Geometry: final body of the model. Coordinates: model frame, mm. Face numbers are marked on the shaded views. A direction names the side the tool comes from. Give positions to 0.01 mm unless a question says otherwise; leave off trailing zeros. Write each loop counter-clockwise with the first axis right and the second up, starting at its lowest first coordinate (ties: lowest second). Pieces come first, ordered by that corner, then holes. Notation, with made-up numbers: (67.25, -34.75) -> (122.25, -34.75) arc R19 cw to (122.25, -14.75) -> close; hole circle Ø5 at (57, 22). An arc over 180 degrees is marked (long way). Answer in a Markdown table with one row per item. Add a question column.
Item 1: Section query B-B on z = 33. Output: boundary loops of the cut face in (x, y).
Item 2: Access query for the marked faces 1, 2 and 3. Directions: +Z, -Z, +X, -X, +Y, -Y. A direction counts if a zero-diameter tool reaches every point of the face in a straight line with its end or side. Return the directions, or none.
Item 3: Section query D-D on z = -75.5. Output: boundary loops of the cut face in (x, y), plus the area to 3 significant figures.
Item 4: Section query A-A on x = 117. Output: boundary loops of the cut face in (y, z).
Item 5: Material intervals for probe 1 along Z at (x, y) = (72, 23); probe 2 along X at (y, z) = (17.5, -63); probe 3 along Y at (x, z) = (-121.5, -13), sorted ascending. Write a range as from..to.
Item 6: First-contact query: P1, Ø10, axis at y = 18.5, z = -2, coming from the +X side; P2, Ø5, axis at y = 19.5, z = -35, coming from the +X side; P3, Ø10, axis at y = 13, z = -11.5, coming from the -X side. Flat tips, straight axial feed; report the tip coordinate or a pass-through.
Item 7: Section query C-C on y = 13.5. State how many separate pieces and enclosed holes the cut face has, plus the area to 3 significant figures.
```python
from build123d import *

# Parameters (mm, degrees)
BOSS_EXTRUDE1_DEPTH = 5
SKETCH2_W           = 71.143127042
SKETCH2_H           = 10
BOSS_EXTRUDE3_DEPTH = 25
SKETCH3_W           = 10
SKETCH3_H           = 10
BOSS_EXTRUDE4_DEPTH = 25
BOSS_EXTRUDE5_DEPTH = 10
SKETCH6_W           = 10
SKETCH6_H           = 60
BOSS_EXTRUDE6_DEPTH = 25
BOSS_EXTRUDE7_DEPTH = 10
SKETCH9_W           = 97.713745916
SKETCH9_H           = 10
BOSS_EXTRUDE8_DEPTH = 25
SKETCH11_R          = 2.5
CUT_EXTRUDE1_DEPTH  = 5
SKETCH12_R          = 1.788924299
CUT_EXTRUDE2_DEPTH  = 10


with BuildPart() as part:
    # Sketch1 → Boss-Extrude1 (new body)
    with BuildSketch(Plane(origin=(0, 0, 0), x_dir=(1, 0, 0), z_dir=(0, 1, 0))):
        with BuildLine():
            Line((-130, 90), (130, 90))
            ThreePointArc((130, 90), (151.213203436, 81.213203436), (160, 60))
            Line((160, 60), (160, -60))
            ThreePointArc((160, -60), (151.213203436, -81.213203436), (130, -90))
            Line((130, -90), (-130, -90))
            ThreePointArc((-130, -90), (-151.213203436, -81.213203436), (-160, -60))
            Line((-160, -60), (-160, 60))
            ThreePointArc((-160, 60), (-151.213203436, 81.213203436), (-130, 90))
        make_face()
    extrude(amount=BOSS_EXTRUDE1_DEPTH)

    # Sketch2 → Boss-Extrude3 (add)
    with BuildSketch(Plane(origin=(0, 5, 0), x_dir=(1, 0, 0), z_dir=(0, 1, 0))):
        with Locations((-84.428436479, 65)):
            Rectangle(SKETCH2_W, SKETCH2_H)
        with Locations((84.428436479, 65)):
            Rectangle(SKETCH2_W, SKETCH2_H)
        with Locations((84.428436479, -65)):
            Rectangle(SKETCH2_W, SKETCH2_H)
        with Locations((-84.428436479, -65)):
            Rectangle(SKETCH2_W, SKETCH2_H)
    extrude(amount=BOSS_EXTRUDE3_DEPTH)

    # Sketch3 → Boss-Extrude4 (add)
    with BuildSketch(Plane(origin=(0, 5, 0), x_dir=(1, 0, 0), z_dir=(0, 1, 0))):
        with Locations((-140, -5)):
            Rectangle(SKETCH3_W, SKETCH3_H)
    boss_extrude4 = extrude(amount=BOSS_EXTRUDE4_DEPTH)

    # Sketch5 → Boss-Extrude5 (add)
    with BuildSketch(Plane(origin=(0, 0, 0), x_dir=(-1, 0, 0), z_dir=(0, 0, -1))):
        Polygon((145, 5), (145, 30), (160, 5), align=None)
    boss_extrude5 = extrude(amount=-BOSS_EXTRUDE5_DEPTH)

    # Sketch6 → Boss-Extrude6 (add)
    with BuildSketch(Plane(origin=(0, 5, 0), x_dir=(1, 0, 0), z_dir=(0, 1, 0))):
        with Locations((70, 0)):
            Rectangle(SKETCH6_W, SKETCH6_H)
    extrude(amount=BOSS_EXTRUDE6_DEPTH)

    # Sketch8 → Boss-Extrude7 (add)
    with BuildSketch(Plane.XY.offset(30)):
        Polygon((75, 30), (88.085238775, 5), (75, 5), align=None)
    boss_extrude7 = extrude(amount=-BOSS_EXTRUDE7_DEPTH)

    # Mirror1: Boss-Extrude7 across plane
    add(boss_extrude7.mirror(Plane(origin=(0, 0, 0), x_dir=(1, 0, 0), z_dir=(0, 0, -1))))

    # Mirror2: Boss-Extrude4, Boss-Extrude5 across plane
    add(boss_extrude4.mirror(Plane(origin=(-145, 30, 0), x_dir=(1, 0, 0), z_dir=(0, 0, 1))))
    add(boss_extrude5.mirror(Plane(origin=(-145, 30, 0), x_dir=(1, 0, 0), z_dir=(0, 0, 1))))

    # Sketch9 → Boss-Extrude8 (add)
    with BuildSketch(Plane(origin=(0, 5, 0), x_dir=(1, 0, 0), z_dir=(0, 1, 0))):
        with Locations((0, -35)):
            Rectangle(SKETCH9_W, SKETCH9_H)
    boss_extrude8 = extrude(amount=BOSS_EXTRUDE8_DEPTH)

    # Mirror3: Boss-Extrude8 across plane
    add(boss_extrude8.mirror(Plane(origin=(0, 0, 0), x_dir=(1, 0, 0), z_dir=(0, 0, -1))))

    # Sketch11 → Cut-Extrude1 (cut)
    with BuildSketch(Plane(origin=(0, 5, 0), x_dir=(1, 0, 0), z_dir=(0, 1, 0))):
        with Locations(Location((-118.275690488, 50, 0), (0, 0, 270))):
            Circle(SKETCH11_R)
        with Locations(Location((-118.275690488, -50, 0), (0, 0, 270))):
            Circle(SKETCH11_R)
        with Locations(Location((20.561944572, -50, 0), (0, 0, 270))):
            Circle(SKETCH11_R)
        with Locations(Location((20.561944572, 50, 0), (0, 0, 270))):
            Circle(SKETCH11_R)
    extrude(amount=-CUT_EXTRUDE1_DEPTH, mode=Mode.SUBTRACT)

    # Sketch12 → Cut-Extrude2 (cut)
    with BuildSketch(Plane.XY.offset(70)):
        with Locations((-58.856872958, 27)):
            Circle(SKETCH12_R)
        with Locations(Location((-58.856872958, 8, 0), (0, 0, 180))):
            Circle(SKETCH12_R)
        with Locations((58.856872958, 8)):
            Circle(SKETCH12_R)
        with Locations(Location((58.856872958, 27, 0), (0, 0, 180))):
            Circle(SKETCH12_R)
    cut_extrude2 = extrude(amount=-CUT_EXTRUDE2_DEPTH, mode=Mode.SUBTRACT)

    # Mirror4: Cut-Extrude2 across plane
    add(cut_extrude2.mirror(Plane.XY), mode=Mode.SUBTRACT)


solid = part.part
```
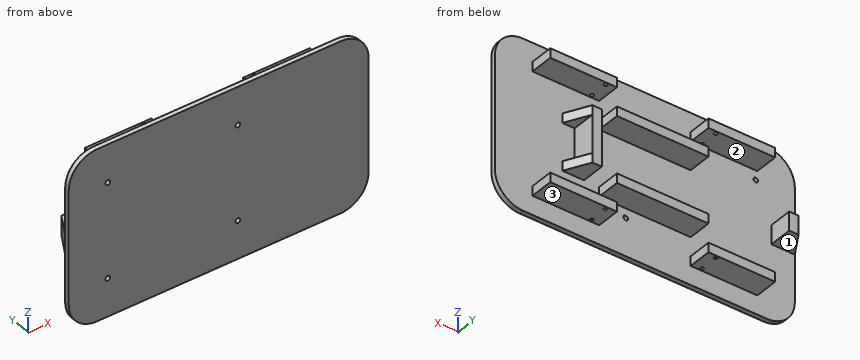
Findings below:
| question | item | result |
|---|---|---|
| 1 | outline | (-160, 0) -> (160, 0) -> (160, 5) -> (48.86, 5) -> (48.86, 30) -> (-48.86, 30) -> (-48.86, 5) -> (-160, 5) -> close |
| 2 | face 1 | -Z, -X, +Y |
| 2 | face 2 | +X, -X, +Y |
| 2 | face 3 | -Z, +X, -X, +Y |
| 3 | outline | (-155.69, 0) -> (155.69, 0) -> (155.69, 5) -> (-155.69, 5) -> close |
| 3 | area | 1,560 mm^2 |
| 4 | outline | (0, -90) -> (5, -90) -> (5, -70) -> (30, -70) -> (30, -60) -> (5, -60) -> (5, 60) -> (30, 60) -> (30, 70) -> (5, 70) -> (5, 90) -> (0, 90) -> close |
| 5 | probe 1 | z = -70..-60, -30..30, 60..70 |
| 5 | probe 2 | x = -120..-48.86, 48.86..120 |
| 5 | probe 3 | y = 0..5 |
| 6 | P1 | stops at x = 75 |
| 6 | P2 | stops at x = 48.86 |
| 6 | P3 | stops at x = -158.06 |
| 7 | separate pieces | 8 |
| 7 | enclosed holes | 0 |
| 7 | area | 5,970 mm^2 |
